Read the model definition and answer for the solid it produces. Units are mm, in the model's axes. A direction names the side the tool comes from. Coordinates: 2 decimals unless noted, no trailing zeros. Loops run counter-clockwise (first coordinate to the right, second up) from the corner with the lowest first, then second, coordinate; pieces in that order, holes last. Notation, with made-up numbers: (59, 38) -> (69, 38) arc R23 ccw to (69, 71) -> close; hole circle Ø3 at (-29, 0.5). An arc over 180 degrees is marked (long way). Answer as a JSON object with one key per item and string values. Group by question number.
Q1. Determine the mould class of faces 1 (the flat face through (-16.25, 15.2, 16.6)), 2 (the flat face through (-18, -16.5, 19)), 3 (the flat face through (0, -16, 0)) for opening direction Z: released by +Z, released by -Z, zero draft, split by the parting line, or undercut.
Q2. Each of these flat-tipped pins is pushed along its axis until it touches: P1, Ø1.5, axis at x = 7, y = 2.5, coming from the +Z side; P2, Ø6, axis at x = -8, y = -13.5, coming from the +Z side; P3, Ø1, axis at y = -10, z = 3, coming from the -X side. Where does it stop, or does it pass through?
Q3. The part is cut by section A-A on y = -3.5. Write down the section's boundary in (x, z) (3 decimals), and give its area (3 significant figures).
Q4. The part is cut by section D-D on z = 35. Write down the section's boundary in (x, y).
Q5. The part is cut by section B-B on z = 13. Write down the section's boundary in (x, y), and give its area (3 significant figures).
Q6. The part is cut by section C-C on x = 12.5. Write down the section's boundary in (y, z) (3 decimals), and give its area (3 significant figures).
Q7. For faces 4 (the flat face through (15.264, -12.711, 31.902)), 5 (the flat face through (-19.25, -15, 19)), 6 (the flat face through (0, 1, 2.65)), 7 (the flat face through (0, 1, 35.65)), determine the directions among +Z, -Z, +X, -X, +Y, -Y from which every point of the face is accessible in a straight line to the end or side of a thin tool.
Q8. Straight lines are drawn through the part: line 1 along Z through (x, y) = (-4, -13.5) (3 decimals); line 2 along Y through (x, z) = (-1.5, 19); line 3 along Z through (x, y) = (-8, -16.5). For each, find the intervals that lie inside material, in ascending order. Write a range as [from, to].
from build123d import *

# Parameters (mm, degrees)
SKETCH1_W                = 30
SKETCH1_H                = 29
SKETCH1_R                = 1.75
BOSS_EXTRUDE1_DEPTH      = 2
SKETCH2_W                = 43.8
SKETCH2_H                = 38.3
BOSS_EXTRUDE3_DEPTH      = 9
BOSS_EXTRUDE4_DEPTH      = 43.8
SKETCH16_W               = 2
SKETCH16_H               = 29
CUT_EXTRUDE1_DEPTH       = 26.5
SKETCH15_W               = 32.5
SKETCH15_H               = 31.5
BOSS_EXTRUDE5_DEPTH      = 2
BOSS_EXTRUDE5_DEPTH_BACK = 31
SKETCH20_W               = 29.25
SKETCH20_H               = 29.5
CUT_EXTRUDE2_DEPTH       = 22.9
CUT_EXTRUDE2_DEPTH_BACK  = 22.9
BOSS_EXTRUDE6_DEPTH      = 2
SKETCH22_W               = 3
SKETCH22_H               = 29.25
CUT_EXTRUDE3_DEPTH       = 2


with BuildPart() as part:
    # Sketch1 → Boss-Extrude1 (new body)
    with BuildSketch(Plane.XY):
        Rectangle(SKETCH1_W, SKETCH1_H)
        with Locations((-8.45, 8.168333333)):
            Circle(SKETCH1_R, mode=Mode.SUBTRACT)
        with Locations((8.168333333, 8.45)):
            Circle(SKETCH1_R, mode=Mode.SUBTRACT)
        with Locations((8.45, -8.168333333)):
            Circle(SKETCH1_R, mode=Mode.SUBTRACT)
        with Locations((-8.168333333, -8.45)):
            Circle(SKETCH1_R, mode=Mode.SUBTRACT)
    extrude(amount=BOSS_EXTRUDE1_DEPTH)

    # Sketch2 → Boss-Extrude3 (add)
    with BuildSketch(Plane.XZ.offset(14.5)):
        with Locations((0, 19.15)):
            Rectangle(SKETCH2_W, SKETCH2_H)
    extrude(amount=BOSS_EXTRUDE3_DEPTH)

    # Sketch3 → Boss-Extrude4 (add)
    with BuildSketch(Plane.ZY.offset(21.9)):
        Polygon((0, -23.5), (-2.5, -23.5), (0, -16.6), align=None)
        Polygon((38.3, -23.5), (40.8, -23.5), (38.3, -16.6), align=None)
    extrude(amount=-BOSS_EXTRUDE4_DEPTH)

    # Sketch16 → Cut-Extrude1 (cut, symmetric)
    with BuildSketch(Plane(origin=(0, 0, 0), x_dir=(0, 0, -1), z_dir=(1, 0, 0))):
        with Locations((-1, 0)):
            Rectangle(SKETCH16_W, SKETCH16_H)
    extrude(amount=CUT_EXTRUDE1_DEPTH, both=True, mode=Mode.SUBTRACT)

    # Sketch15 → Boss-Extrude5 (add, two sides)
    with BuildSketch(Plane(origin=(0, 0, 4.65), x_dir=(-1, 0, 0), z_dir=(0, 0, -1))) as boss_extrude5_sk:
        with Locations((0, 1.25)):
            Rectangle(SKETCH15_W, SKETCH15_H)
    extrude(amount=BOSS_EXTRUDE5_DEPTH)
    extrude(boss_extrude5_sk.sketch, amount=-BOSS_EXTRUDE5_DEPTH_BACK)

    # Sketch20 → Cut-Extrude2 (cut, two sides)
    with BuildSketch(Plane(origin=(0, 0, 0), x_dir=(0, 0, -1), z_dir=(1, 0, 0))) as cut_extrude2_sk:
        with Locations((-19.15, 0.25)):
            Rectangle(SKETCH20_W, SKETCH20_H)
    extrude(amount=CUT_EXTRUDE2_DEPTH, mode=Mode.SUBTRACT)
    extrude(cut_extrude2_sk.sketch, amount=-CUT_EXTRUDE2_DEPTH_BACK, mode=Mode.SUBTRACT)

    # Sketch21 → Boss-Extrude6 (add)
    with BuildSketch(Plane(origin=(16.25, 0, 0), x_dir=(0, 0, -1), z_dir=(1, 0, 0))):
        Polygon((-35.65, -10.971015683), (-33.775, -10.971015683), (-29.976700434, -14.5), (-35.65, -14.5), align=None)
        Polygon((-4.525, -10.971015683), (-8.323299566, -14.5), (-2.65, -14.5), (-2.65, -10.971015683), align=None)
    extrude(amount=-BOSS_EXTRUDE6_DEPTH)

    # Sketch22 → Cut-Extrude3 (cut)
    with BuildSketch(Plane(origin=(0, -14.5, 0), x_dir=(1, 0, 0), z_dir=(0, 1, 0))):
        with Locations((-17.75, -19.15)):
            Rectangle(SKETCH22_W, SKETCH22_H)
    extrude(amount=-CUT_EXTRUDE3_DEPTH, mode=Mode.SUBTRACT)


solid = part.part
Final values:
{
 "1": {"face 1": "zero draft", "face 2": "undercut", "face 3": "released by -Z"},
 "2": {"P1": "stops at z = 35.65", "P2": "stops at z = 38.3", "P3": "stops at x = -16.25"},
 "3": {"outline": "(-16.25, 2.65) -> (16.25, 2.65) -> (16.25, 4.525) -> (-16.25, 4.525) -> close; (-16.25, 33.775) -> (16.25, 33.775) -> (16.25, 35.65) -> (-16.25, 35.65) -> close", "area": "122 mm2"},
 "4": {"outline": "(-21.9, -23.5) -> (21.9, -23.5) -> (21.9, -14.5) -> (16.25, -14.5) -> (16.25, 17) -> (-16.25, 17) -> (-16.25, -14.5) -> (-21.9, -14.5) -> close"},
 "5": {"outline": "(-21.9, -23.5) -> (21.9, -23.5) -> (21.9, -14.5) -> (-16.25, -14.5) -> (-16.25, -16.5) -> (-19.25, -16.5) -> (-19.25, -14.5) -> (-21.9, -14.5) -> close; (-16.25, 15) -> (16.25, 15) -> (16.25, 17) -> (-16.25, 17) -> close", "area": "453 mm2"},
 "6": {"outline": "(-23.5, -2.5) -> (-16.6, 0) -> (-14.5, 0) -> (-14.5, 2.65) -> (17, 2.65) -> (17, 35.65) -> (-14.5, 35.65) -> (-14.5, 38.3) -> (-16.6, 38.3) -> (-23.5, 40.8) -> close; hole (-14.5, 4.525) -> (15, 4.525) -> (15, 33.775) -> (-14.5, 33.775) -> close", "area": "539 mm2"},
 "7": {"face 4": "+X, -X", "face 5": "+Y", "face 6": "-Z, +X, -X, +Y", "face 7": "+Z, +X, -X, +Y"},
 "8": {"line 1": "z = [2.65, 4.525], [33.775, 35.65]", "line 2": "y = [-23.5, -14.5], [15, 17]", "line 3": "z = [0, 38.3]"}
}
